The drawing under review shows one solid part. Ordinate dimensions are in mm from its lowest x, y, z. A direction names the side the tool comes from. Coordinates: 2 decimals unless noted, no trailing zeros. Order: outer loops, then holes, each group sorted by start corner. A loop starts at its lowest first (then second) coordinate and runs counter-clockwise, first axis right, second up. Notation, with made-up numbers: (30, -16.75) -> (68, -16.75) arc R32 ccw to (68, 17.25) -> close; hole circle Ø2 at (-36.5, 65.25). An arc over 180 degrees is marked (long way). Put each result on its own line as item: value.
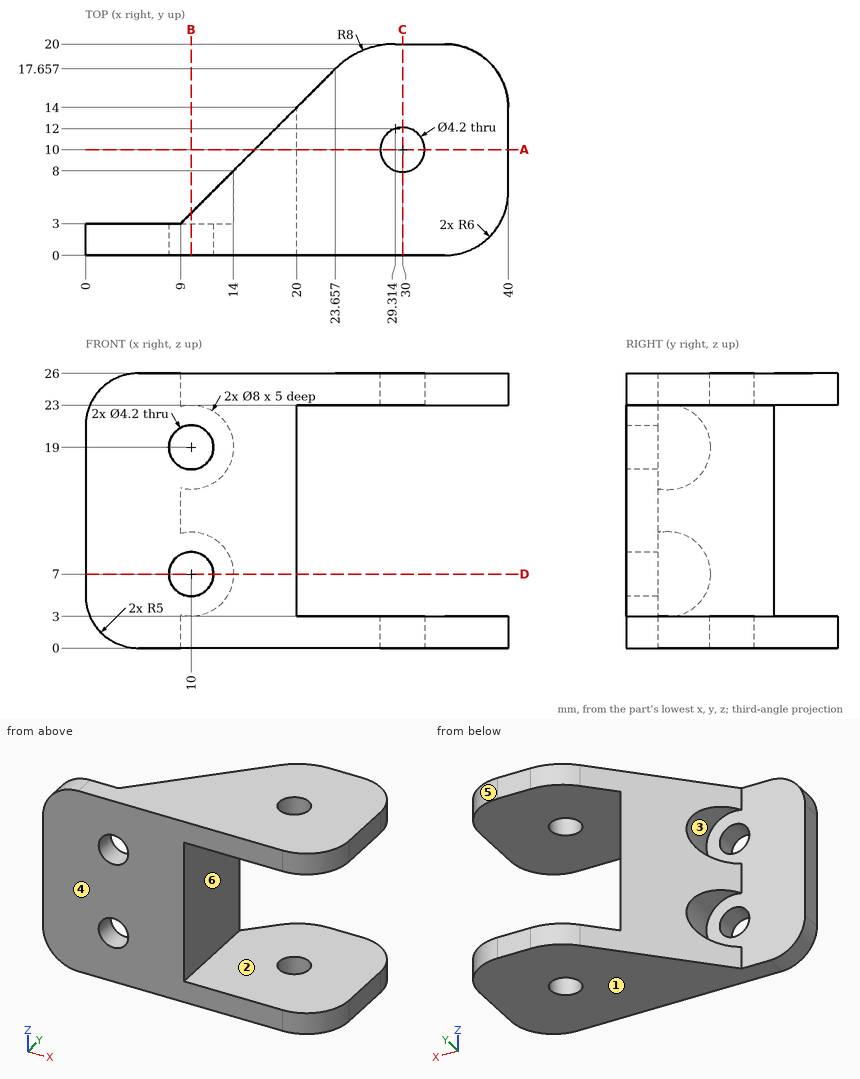
Item 1: For the marked faces 5 and 6, list the 3-axis set-ups (+Z, -Z, +X, -X, +Y, -Y) from which the entire face can be reached by the end or side of a thin tool; tool diameter is ignored.
Answers below:
face 5: +Z, -Z, +X, +Y
face 6: +X, +Y, -Y
Item 2: Consider section C-C on x = 30. Write out the cut boundary in (y, z).
Answers below:
outline: (0, 0) -> (7.9, 0) -> (7.9, 3) -> (0, 3) -> close; (0, 23) -> (7.9, 23) -> (7.9, 26) -> (0, 26) -> close; (12.1, 0) -> (20, 0) -> (20, 3) -> (12.1, 3) -> close; (12.1, 23) -> (20, 23) -> (20, 26) -> (12.1, 26) -> close
Item 3: For pin 1 Ø13 at (x, z) = (10, 7) entering from -Y; pin 2 Ø7 at (y, z) = (4.5, 16) entering from +X; pin 3 Ø3 at (y, z) = (9.5, 10.5) entering from -X; pin 4 Ø5 at (x, z) = (10, 19) entering from +Y, all flat-tipped, find the tip position at first contact; note any pin that passes through.
Answers below:
pin 1: y = 0
pin 2: x = 20
pin 3: x = 14
pin 4: y = 3
Item 4: Consider section A-A on y = 10. Write out the cut boundary in (x, z), and give its area (3 significant figures).
Answers below:
outline: (16, 0) -> (27.9, 0) -> (27.9, 3) -> (20, 3) -> (20, 23) -> (27.9, 23) -> (27.9, 26) -> (16, 26) -> close; (32.1, 0) -> (40, 0) -> (40, 3) -> (32.1, 3) -> close; (32.1, 23) -> (40, 23) -> (40, 26) -> (32.1, 26) -> close
area: 199 mm^2
Item 5: For line 1 (Z direction, x = 33.5, y = 9); line 2 (X direction, y = 4.9, z = 19); line 3 (Y direction, x = 10.5, z = 22.5), list the stretches that pass through material, from the lowest coordinate up. Write a range as from..to.
Answers below:
line 1: 0..3, 23..26
line 2: 14..20
line 3: 0..3
Item 6: Mouldability with a two-part tool opening along Z and no side actions: class the marked faces 1, 2, 3 and 4 as +Z half, -Z half, draft (parallel to the pull), parting line (faces both ways), or undercut.
Answers below:
face 1: -Z half
face 2: undercut
face 3: undercut
face 4: draft
Item 7: Consider section B-B on x = 10. Write out the cut boundary in (y, z), and give its area (3 significant figures).
Answers below:
outline: (0, 0) -> (4, 0) -> (4, 3) -> (3, 3) -> (3, 4.9) -> (0, 4.9) -> close; (0, 9.1) -> (3, 9.1) -> (3, 11) -> (4, 11) -> (4, 15) -> (3, 15) -> (3, 16.9) -> (0, 16.9) -> close; (0, 21.1) -> (3, 21.1) -> (3, 23) -> (4, 23) -> (4, 26) -> (0, 26) -> close
area: 62.8 mm^2
Item 8: Consider section D-D on z = 7. Write out the cut boundary in (x, y), and give its area (3 significant figures).
Answers below:
outline: (0, 0) -> (7.9, 0) -> (7.9, 3) -> (0, 3) -> close; (12.1, 0) -> (20, 0) -> (20, 14) -> (14, 8) -> (14, 3) -> (12.1, 3) -> close
area: 95.4 mm^2
